For this review, take the finished solid that the model builds, in its own axes (mm). Face numbers are marked on the shaded views. A direction names the side the tool comes from. Give positions to 0.01 mm unless a question says otherwise; leave off trailing zeros. Order: outer loops, then holes, each group sorted by start corner. A loop starts at its lowest first (then second) coordinate and runs counter-clockwise, first axis right, second up.
from build123d import *

# Parameters (mm, degrees)
BOSS_EXTRUDE1_DEPTH        = 50
BOSS_EXTRUDE3_DEPTH        = 55
BOSS_EXTRUDE4_DEPTH        = 25
BOSS_EXTRUDE5_DEPTH        = 7.5
M16X1_5_TAPPED_HOLE1_D     = 14.5
M16X1_5_TAPPED_HOLE1_DEPTH = 20.643760512
M16X1_5_TAPPED_HOLE1_TIP   = 4.356239488
SKETCH7_R                  = 25
SKETCH7_R_2                = 10
BOSS_EXTRUDE6_DEPTH        = 2.5
SKETCH7_2_R                = 10
CUT_EXTRUDE1_DEPTH         = 421.386726717
SKETCH8_W                  = 60
SKETCH8_H                  = 8
CUT_EXTRUDE2_DEPTH         = 434.416658655
FILLET1_R                  = 20
FILLET2_R                  = 10
FILLET3_R                  = 10
FILLET4_R                  = 13
FILLET5_R                  = 25


with BuildPart() as part:
    # Sketch2 → Boss-Extrude1 (new, symmetric)
    with BuildSketch(Plane(origin=(0, 0, 0), x_dir=(0, 0, -1), z_dir=(1, 0, 0))):
        Polygon((-25, 245), (-25, 225), (-25, 0), (0, 0), (0, 360), (-25, 360), (-25, 250), align=None)
        with BuildLine():
            ThreePointArc((-95, 245), (-96.054684353, 234.784517816), (-99.17424305, 225))
            Line((-99.17424305, 225), (-25, 225))
            Line((-25, 225), (-25, 245))
            Line((-25, 245), (-95, 245))
        make_face()
        with BuildLine():
            ThreePointArc((-95.250628145, 250), (-95.062696344, 247.503138753), (-95, 245))
            Line((-95, 245), (-25, 245))
            Line((-25, 245), (-25, 250))
            Line((-25, 250), (-95.250628145, 250))
        make_face()
        with BuildLine():
            ThreePointArc((-190.82575695, 225), (-193.945315647, 234.784517816), (-195, 245))
            Line((-195, 245), (-235, 245))
            Line((-235, 245), (-235, 225))
            Line((-235, 225), (-190.82575695, 225))
        make_face()
        with BuildLine():
            Line((-235, 245), (-195, 245))
            ThreePointArc((-195, 245), (-194.937303656, 247.503138753), (-194.749371855, 250))
            Line((-194.749371855, 250), (-235, 250))
            Line((-235, 250), (-235, 245))
        make_face()
    extrude(amount=BOSS_EXTRUDE1_DEPTH, both=True)

    # Sketch2_3 → Boss-Extrude3 (add, symmetric)
    with BuildSketch(Plane(origin=(0, 0, 0), x_dir=(0, 0, -1), z_dir=(1, 0, 0))):
        with BuildLine():
            Line((-185, 245), (-190, 245))
            Line((-190, 245), (-190, 250))
            Line((-190, 250), (-194.749371855, 250))
            ThreePointArc((-194.749371855, 250), (-145, 195), (-95.250628145, 250))
            Line((-95.250628145, 250), (-100, 250))
            Line((-100, 250), (-100, 245))
            Line((-100, 245), (-105, 245))
            ThreePointArc((-105, 245), (-145, 205), (-185, 245))
        make_face()
    extrude(amount=BOSS_EXTRUDE3_DEPTH, both=True)

    # Sketch4 → Boss-Extrude4 (add, symmetric)
    with BuildSketch(Plane(origin=(0, 0, 0), x_dir=(0, 0, -1), z_dir=(1, 0, 0))):
        with BuildLine():
            Line((-175.781812899, 140.427664129), (-25, 85.547572365))
            Line((-25, 85.547572365), (-25, 96.18935009))
            Line((-25, 96.18935009), (-172.361611466, 149.824590337))
            ThreePointArc((-172.361611466, 149.824590337), (-210.532163543, 179.113885092), (-225, 225))
            Line((-225, 225), (-235, 225))
            ThreePointArc((-235, 225), (-218.723683986, 173.378120728), (-175.781812899, 140.427664129))
        make_face()
    extrude(amount=BOSS_EXTRUDE4_DEPTH, both=True)

    # Sketch4_3 → Boss-Extrude5 (add, symmetric)
    with BuildSketch(Plane(origin=(0, 0, 0), x_dir=(0, 0, -1), z_dir=(1, 0, 0))):
        with BuildLine():
            Line((-172.361611466, 149.824590337), (-25, 96.18935009))
            Line((-25, 96.18935009), (-25, 225))
            Line((-25, 225), (-99.17424305, 225))
            ThreePointArc((-99.17424305, 225), (-145, 195), (-190.82575695, 225))
            Line((-190.82575695, 225), (-225, 225))
            ThreePointArc((-225, 225), (-210.532163543, 179.113885092), (-172.361611466, 149.824590337))
        make_face()
    extrude(amount=BOSS_EXTRUDE5_DEPTH, both=True)

    # M16x1.5 Tapped Hole1
    with Locations(Plane(origin=(0, 250, 0), x_dir=(1, 0, 0), z_dir=(0, 1, 0))):
        with Locations((0, -215), (0, -75)):
            Hole(M16X1_5_TAPPED_HOLE1_D / 2, depth=M16X1_5_TAPPED_HOLE1_DEPTH)
            with Locations((0, 0, -(M16X1_5_TAPPED_HOLE1_DEPTH + M16X1_5_TAPPED_HOLE1_TIP / 2))):  # 118° drill point
                Cone(0, M16X1_5_TAPPED_HOLE1_D / 2, M16X1_5_TAPPED_HOLE1_TIP, mode=Mode.SUBTRACT)

    # Sketch7 → Boss-Extrude6 (add, symmetric)
    # profile 1 of 2: a face of its own
    with BuildSketch(Plane.XY.offset(25)):
        with Locations((0, 325)):
            Circle(SKETCH7_R)
        with Locations((0, 325)):
            Circle(SKETCH7_R_2, mode=Mode.SUBTRACT)
    # profile 2 of 2: a face of its own
    with BuildSketch(Plane.XY.offset(25)):
        with Locations((0, 35)):
            Circle(SKETCH7_R)
        with Locations((0, 35)):
            Circle(SKETCH7_R_2, mode=Mode.SUBTRACT)
    extrude(amount=BOSS_EXTRUDE6_DEPTH, both=True)

    # Sketch7_2 → Cut-Extrude1 (cut, through all)
    with BuildSketch(Plane.XY.offset(25)):
        with Locations((0, 325)):
            Circle(SKETCH7_2_R)
        with Locations((0, 35)):
            Circle(SKETCH7_2_R)
    extrude(amount=-CUT_EXTRUDE1_DEPTH, mode=Mode.SUBTRACT)

    # Sketch8 → Cut-Extrude2 (cut, through all)
    with BuildSketch(Plane.XZ):
        with Locations((0, 4)):
            Rectangle(SKETCH8_W, SKETCH8_H)
    extrude(amount=-CUT_EXTRUDE2_DEPTH, mode=Mode.SUBTRACT)

    # Fillet1
    fillet1_edges = [part.edges().sort_by_distance(p)[0] for p in [
        (28.75, 225, 25),
        (0, 250, 25),
        (-28.75, 225, 25),
    ]]
    fillet(fillet1_edges, radius=FILLET1_R)

    # Fillet2
    fillet2_edges = [part.edges().sort_by_distance(p)[0] for p in [
        (16.25, 225, 225),
    ]]
    fillet(fillet2_edges, radius=FILLET2_R)

    # Fillet3
    fillet3_edges = [part.edges().sort_by_distance(p)[0] for p in [
        (-16.25, 225, 225),
    ]]
    fillet(fillet3_edges, radius=FILLET3_R)

    # Fillet4
    fillet4_edges = [part.edges().sort_by_distance(p)[0] for p in [
        (16.25, 96.18935009, 25),
        (-16.25, 96.18935009, 25),
    ]]
    fillet(fillet4_edges, radius=FILLET4_R)

    # Fillet5
    fillet5_edges = [part.edges().sort_by_distance(p)[0] for p in [
        (0, 85.547572365, 25),
    ]]
    fillet(fillet5_edges, radius=FILLET5_R)


solid = part.part
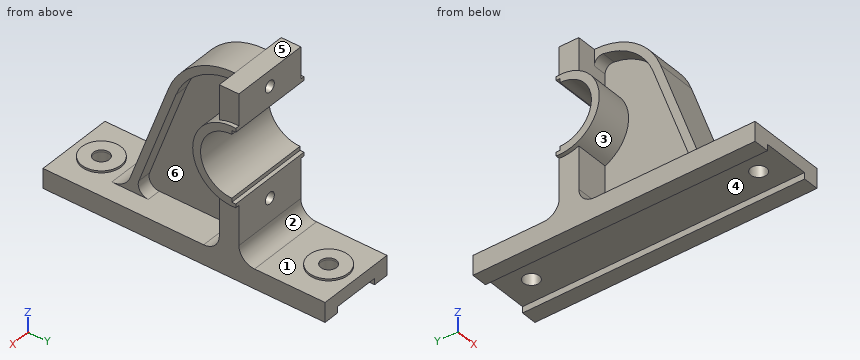
1) Clearance check with flat-ended pins moving along their axes: pin 1 (1 mm diameter, centred on x = -15.5, z = 92, fed in from -Y); pin 2 (8 mm diameter, centred on x = 7.5, z = 58, fed in from +Y); pin 3 (5 mm diameter, centred on x = 7.5, y = 181, fed in from +Z); pin 4 (8 mm diameter, centred on y = 211, z = 133.5, fed in from +X). State where each tip first meets the part, or that it passes through.
Answer sheet:
pin 1: stops at y = 109.75
pin 2: stops at y = 250
pin 3: stops at z = 224.86
pin 4: passes through
2) Tool access review of the marked faces 1, 2 and 3: name each direction out of +Z, -Z, +X, -X, +Y, -Y from which nothing blocks a thin tool from reaching the whole face with its end or side.
Answer sheet:
face 1: +Z
face 2: +Z, +X, -X
face 3: -X
3) We need section B-B on y = 281. Give the boundary of the cut face in (x, z).
Answer sheet:
outline: (-50, 0) - (-30, 0) - (-30, 8) - (30, 8) - (30, 0) - (50, 0) - (50, 25) - (-50, 25) - close
4) We need section C-C on x = 46. Give the boundary of the cut face in (y, z), then the cut area to 3 significant figures.
Answer sheet:
outline: (0, 0) - (360, 0) - (360, 25) - (270, 25) arc R20 cw to (250, 45) - (250, 100) - (245, 100) - (245, 105) arc R40 cw to (245, 185) - (245, 190) - (250, 190) - (250, 235) - (225, 235) - (225, 190.83) arc R50 ccw to (225, 99.17) - (225, 45) arc R20 cw to (205, 25) - (0, 25) - close
area: 13,400 mm2
5) We need section A-A on y = 325. Give the boundary of the cut face in (x, z), then the cut area to 4 significant figures.
Answer sheet:
outline: (-50, 0) - (-30, 0) - (-30, 8) - (-10, 8) - (-10, 27.5) - (-25, 27.5) - (-25, 25) - (-50, 25) - close; (10, 8) - (30, 8) - (30, 0) - (50, 0) - (50, 25) - (25, 25) - (25, 27.5) - (10, 27.5) - close
area: 1,755 mm2
6) To check wall thickness, follow line 1 (Y direction, x = 0, z = 12); line 2 (X direction, y = 237, z = 215); line 3 (X direction, y = 35, z = 20). State the ranges of each line that lie inside material, in increasing order.
Answer sheet:
line 1: y = 0 to 25, 45 to 315, 335 to 360
line 2: x = -50 to -7.25, 7.25 to 50
line 3: x = -50 to -10, 10 to 50
7) Draft analysis for pull direction Z (two halves, no side actions). For the marked faces 4, 5 and 6, state which applies: +Z half, -Z half, draft (parallel to the pull), parting line (faces both ways), or undercut.
Answer sheet:
face 4: -Z half
face 5: +Z half
face 6: undercut
8) We need section D-D on z = 145. Give the boundary of the cut face in (x, y), then the cut area to 3 significant figures.
Answer sheet:
outline: (-55, 195) - (-7.5, 195) - (-7.5, 139.87) - (-25, 139.87) - (-25, 129.22) - (25, 129.22) - (25, 139.87) - (7.5, 139.87) - (7.5, 195) - (55, 195) - (55, 205) - (-55, 205) - close
area: 2,460 mm2
